from build123d import *

# Parameters (mm, degrees)
SKETCH_1_R      = 37.5
SKETCH_1_R_2    = 25
EXTRUDE_1_DEPTH = 2
SKETCH_2_R      = 37.5
SKETCH_2_R_2    = 17.5
EXTRUDE_2_DEPTH = 0.6
SKETCH_3_R      = 37.5
SKETCH_3_R_2    = 17.5
SKETCH_3_R_3    = 4
EXTRUDE_3_DEPTH = 3


with BuildPart() as part:
    # Эскиз1 → Бобышка-Вытянуть1 (new body)
    with BuildSketch(Plane.XY):
        Circle(SKETCH_1_R)
        Circle(SKETCH_1_R_2, mode=Mode.SUBTRACT)
    extrude(amount=EXTRUDE_1_DEPTH)

    # Эскиз2 → Бобышка-Вытянуть2 (add)
    with BuildSketch(Plane.XY.offset(2)):
        Circle(SKETCH_2_R)
        Circle(SKETCH_2_R_2, mode=Mode.SUBTRACT)
    extrude(amount=EXTRUDE_2_DEPTH)

    # Эскиз3 → Бобышка-Вытянуть3 (add)
    with BuildSketch(Plane.XY.offset(2.6)):
        Circle(SKETCH_3_R)
        Circle(SKETCH_3_R_2, mode=Mode.SUBTRACT)
        with Locations((0, 30)):
            Circle(SKETCH_3_R_3, mode=Mode.SUBTRACT)
        with Locations((0, -30)):
            Circle(SKETCH_3_R_3, mode=Mode.SUBTRACT)
        with Locations((30, 0)):
            Circle(SKETCH_3_R_3, mode=Mode.SUBTRACT)
        with Locations((-30, 0)):
            Circle(SKETCH_3_R_3, mode=Mode.SUBTRACT)
        with Locations((23, 21)):
            Circle(SKETCH_3_R_3, mode=Mode.SUBTRACT)
        with Locations((-23, 21)):
            Circle(SKETCH_3_R_3, mode=Mode.SUBTRACT)
        with Locations((-23, -21)):
            Circle(SKETCH_3_R_3, mode=Mode.SUBTRACT)
        with Locations((23, -21)):
            Circle(SKETCH_3_R_3, mode=Mode.SUBTRACT)
    extrude(amount=EXTRUDE_3_DEPTH)


solid = part.part
Check sheet for the modelled part. Datum: model origin and axes. Units: mm. A direction names the side the tool comes from. Round coordinates to 2 decimals unless told otherwise and drop trailing zeros. Loops run counter-clockwise (first coordinate to the right, second up) from the corner with the lowest first, then second, coordinate; pieces in that order, holes last. Notation, with made-up numbers: (36, 16.25) -> (67, 16.25) arc R14 cw to (67, 30.25) -> close; hole circle Ø4 at (4.25, 55.25). An arc over 180 degrees is marked (long way). Put each result on its own line as item: value. Start each with the question number.
1. Draft check along Y on faces 1 (the face through (0, 30, 2.6)), 2 (the face through (8, -16, 5.6)). Enter one of: +Y half, -Y half, draft (parallel to the pull), parting line (faces both ways), or undercut.
2. Section check C-C (z = 3.55). Give the number of separate pieces and of enclosed holes in the cut face, plus the area to 3 significant figures.
3. Scan lines: probe 1 along Y at (x, z) = (-23, 3.4); probe 2 along Y at (x, z) = (-16.5, 0.55); probe 3 along Y at (x, z) = (-22, 1.75). Record each from-to range of solid material in increasing order.
4. Gauge pin test, flat ends, axial feed: pin 1 (8 mm diameter, centred on x = -3, y = 18, fed in from -Z); pin 2 (7 mm diameter, centred on x = -23, y = -21, fed in from +Z); pin 3 (2 mm diameter, centred on x = 23.5, z = 1, fed in from +Y). Record the tip position at first contact, or that the pin passes through.
5. Access from +Z, -Z, +X, -X, +Y, -Y to the whole of each face (thin tool, end or side, straight path). Record for faces 3 (the face through (-17, -5, 2)), 4 (the face through (24, -8, 0)), 5 (the face through (-25.95, -18.3, 4.08)).
6. Section check D-D (x = 30). Enter the section's corners in (y, z), plus the area to 3 significant figures.
7. Section check A-A (x = 0). Enter the section's corners in (y, z), plus the area to 3 significant figures.
Findings:
1. face 1: undercut
1. face 2: draft
2. separate pieces: 1
2. enclosed holes: 9
2. area: 3,050 mm^2
3. probe 1: y = -29.62 to -25, -17 to 17, 25 to 29.62
3. probe 2: y = -33.67 to -18.78, 18.78 to 33.67
3. probe 3: y = -30.37 to -11.87, 11.87 to 30.37
4. pin 1: stops at z = 2
4. pin 2: stops at z = 2.6
4. pin 3: stops at y = 30
5. face 3: -Z
5. face 4: -Z, +X, -X, +Y, -Y
5. face 5: +Z
6. outline: (-22.5, 0) -> (22.5, 0) -> (22.5, 5.6) -> (4, 5.6) -> (4, 2.6) -> (-4, 2.6) -> (-4, 5.6) -> (-22.5, 5.6) -> close
6. area: 228 mm^2
7. outline: (-37.5, 0) -> (-25, 0) -> (-25, 2) -> (-17.5, 2) -> (-17.5, 5.6) -> (-26, 5.6) -> (-26, 2.6) -> (-34, 2.6) -> (-34, 5.6) -> (-37.5, 5.6) -> close; (17.5, 2) -> (25, 2) -> (25, 0) -> (37.5, 0) -> (37.5, 5.6) -> (34, 5.6) -> (34, 2.6) -> (26, 2.6) -> (26, 5.6) -> (17.5, 5.6) -> close
7. area: 146 mm^2
